```python
from build123d import *

# Parameters (mm, degrees)
F1_DEPTH = 63.5
F2_DEPTH = 25.4
F3_DEPTH = 7.9375
F5_R     = 6.35


with BuildPart() as f1:
    # F0 (on Front) → F1 (new body, symmetric)
    with BuildSketch(Plane.XZ):
        Polygon((41.275, -9.525), (41.275, 9.525), (22.225, 9.525), (-41.275, 9.525), (-41.275, -9.525), align=None)
    extrude(amount=F1_DEPTH, both=True)

    # F0 (on Front) → F2 (join, symmetric)
    with BuildSketch(Plane.XZ):
        Polygon((63.9889016747, 62.1188126437), (63.9889016747, 43.0680627667), (85.6312127138, 42.8760321675), (85.8415678118, 61.9249155796), align=None)
        with BuildLine():
            Line((22.225, 9.525), (41.275, 9.525))
            Line((41.275, 9.525), (41.275, 30.394497076))
            ThreePointArc((41.275, 30.394497076), (45.0528398589, 39.4580924516), (54.1495976422, 43.1553661719))
            Line((54.1495976422, 43.1553661719), (63.9889016747, 43.0680627667))
            Line((63.9889016747, 43.0680627667), (63.9889016747, 62.1188126437))
            Line((63.9889016747, 62.1188126437), (54.3186202071, 62.2046163244))
            ThreePointArc((54.3186202071, 62.2046163244), (31.6423473224, 52.9881031659), (22.225, 30.394497076))
            Line((22.225, 30.394497076), (22.225, 9.525))
        make_face()
    extrude(amount=F2_DEPTH, both=True)

    # F0 (on Front) → F3 (join, symmetric)
    with BuildSketch(Plane.XZ):
        with BuildLine():
            Line((-41.275, 9.525), (22.225, 9.525))
            Line((22.225, 9.525), (22.225, 30.394497076))
            ThreePointArc((22.225, 30.394497076), (31.6423473224, 52.9881031659), (54.3186202071, 62.2046163244))
            add(Edge.make_bspline(
                [(-41.275, 9.525), (-32.9198464751, 34.1910012066), (25.594945997, 75.3937736154), (54.3186202071, 62.2046163244)],
                knots=[0, 0, 0, 0, 109.1479830339, 109.1479830339, 109.1479830339, 109.1479830339], degree=3))
        make_face()
    extrude(amount=F3_DEPTH, both=True)

    # F0 (on Front) → F4 (revolve)
    with BuildSketch(Plane.XZ):
        Polygon((85.8415678118, 61.9249155796), (85.6312127138, 42.8760321675), (85.5784714222, 38.1), (114.7889016747, 38.1), (114.7889016747, 66.675), (85.8940225648, 66.675), align=None)
    revolve(axis=Axis((85.7362469935, 0, 52.3875), (0.0110422364, 0, 0.9999390326)))

    # F5
    f5_edges = [f1.edges().sort_by_distance(p)[0] for p in [
        (-41.275, -63.5, 0),
        (41.275, -63.5, 0),
        (41.275, 63.5, 0),
        (-41.275, 63.5, 0),
    ]]
    fillet(f5_edges, radius=F5_R)


solid = f1.part
```
Read the model definition and answer for the solid it produces. Units are mm, in the model's axes. A direction names the side the tool comes from. Round coordinates to 2 decimals unless told otherwise and drop trailing zeros. Write each loop counter-clockwise with the first axis right and the second up, starting at its lowest first coordinate (ties: lowest second). Pieces come first, ordered by that corner, then holes. Notation, with made-up numbers: (65, 19) - (114, 19) arc R22 ccw to (114, 28) - close; hole circle Ø2 at (7, 29). An arc over 180 degrees is marked (long way). Use CSV: the item, a comma, the result in double quotes.
Q1. Find section A-A, the plane z = 4. Write down the section's boundary in (x, y) (3 decimals), then the cut area to 3 significant figures.
Values:
outline,"(-41.275, -57.15) arc R6.35 ccw to (-34.925, -63.5) - (34.925, -63.5) arc R6.35 ccw to (41.275, -57.15) - (41.275, 57.15) arc R6.35 ccw to (34.925, 63.5) - (-34.925, 63.5) arc R6.35 ccw to (-41.275, 57.15) - close"
area,"10,400 mm²"
Q2. Find section B-B, the plane y = 47.5. Write down the section's boundary in (x, z) (3 decimals).
Values:
outline,"(-41.275, -9.525) - (41.275, -9.525) - (41.275, 9.525) - (-41.275, 9.525) - close"
Q3. Straight lines are drawn through the part: line 1 along Z through (x, y) = (-7, -33.5) (3 decimals); line 2 along X through (y, z) = (10, -5) (3 decimals); line 3 along Y through (x, z) = (7, 35). For each, find the intervals that lie inside material, in ascending order.
Values:
line 1,"z = -9.525 to 9.525"
line 2,"x = -41.275 to 41.275"
line 3,"y = -7.94 to 7.94"
Q4. Each of these flat-tipped pins is pushed along its axis until it touches: pin 1 Ø5 at (y, z) = (16, 24) entering from -X (3 decimals); pin 2 Ø1 at (y, z) = (0.5, 49) entering from -X; pin 3 Ø12 at (x, y) = (36, -10.5) entering from +Z. Where does it stop, or does it pass through?
Values:
pin 1,"stops at x = 22.225"
pin 2,"stops at x = -3.62"
pin 3,"stops at z = 64.75"
Q5. A tool of negligible diameter and unlimited length cuts with its end or side. For faces 1 (the flat face through (22.225, -17, 20)), 2 (the cylindrical face through (39.464, 61.59, 0.133)), 3 (the flat face through (22.225, 17, 20)), 4 (the conical face through (87.3, -0.7, 38.1)), 5 (the flat face through (41.275, -1, 6)), from which of +Z, -Z, +X, -X, +Y, -Y can it reach the whole face along a straight path? Write none if from no direction.
Values:
face 1,"+Z, -X, -Y"
face 2,"+Z, -Z, +X, +Y"
face 3,"+Z, -X, +Y"
face 4,"-Z"
face 5,"-Z, +X, +Y, -Y"
Q6. Determine the mould class of faces 6 (the cylindrical face through (-39.365, -61.689, -0.133)), 7 (the conical face through (84.493, 0.062, 66.706)), 8 (the flat face through (0, 63.5, 0)) for opening direction Y: +Y half, -Y half, draft (parallel to the pull), parting line (faces both ways), or undercut.
Values:
face 6,"-Y half"
face 7,"undercut"
face 8,"+Y half"
